Can you work these out from the model? Positions are in its coordinate system, mm. A direction names the side the tool comes from. Coordinates: 2 decimals unless noted, no trailing zeros. Order: outer loops, then holes, each group sorted by start corner. A loop starts at its lowest first (then second) coordinate and runs counter-clockwise, first axis right, second up. Notation, with made-up numbers: (11, 64.5) - (42, 64.5) arc R17 cw to (42, 93.5) - close; hole circle Ø5 at (-9, -8). An arc over 180 degrees is marked (long way). Use a Markdown table: item, result. Add a question column.
(1) I want a section at D-D (x = -2). List the corners of the cut face in (y, z) for me, and give its area (3 significant figures).
(2) I want a section at B-B (z = 1.3). List the corners of the cut face in (x, y) for me, and give its area (3 significant figures).
(3) We'd pull the mould along Y, two halves only. Please class faces 1 (the flat face through (30, 0, 2)), 2 (the cylindrical face through (-18.4, 1.2, 2.5)), 3 (the cylindrical face through (-3.45, 10.88, 2.54)): pulls with the +Y half, pulls with the -Y half, needs draft (parallel to the pull), parting line crosses it, or undercut.
(4) For pin 1 Ø5 at (x, y) = (-20, 0) entering from -Z, with a flat end and sliding along its axis, tell me the tip position at first contact or that it passes through.
(5) On a 3-axis mill with a long thin cutter (end or side, diameter ignored), from which of +Z, -Z, +X, -X, +Y, -Y can I reach the whole of each face in a straight line? I mean faces 4 (the flat face through (6, -15, 2)), 5 (the cylindrical face through (28, -19, 3)), 6 (the flat face through (6, 15, 2)). Say none if no direction works.
(6) I want a section at C-C (y = 0). List the corners of the cut face in (x, z) for me.
(7) If I drill on L1, parallel to Y at x = 20, z = 2.35; L2, parallel to X at y = -1, z = 1.2; L3, parallel to X at y = -1.5, z = 2.65, over which ranges is the centre line in solid material (lowest first)? Write a range as [from, to].
(8) I want a section at A-A (x = -20). List the corners of the cut face in (y, z) for me.
```python
from build123d import *

# Parameters (mm, degrees)
ESQUISSE1_R        = 2
BOSS_EXTRU_1_DEPTH = 5
CONG_1_R           = 5


with BuildPart() as part:
    # Esquisse1 → Boss.-Extru.1 (new body)
    with BuildSketch(Plane.XY):
        Polygon((-30, 20), (-30, -20), (-8, -20), (-4, -10), (4, -10), (8, -20), (30, -20), (30, 20), (8, 20), (4, 10), (-4, 10), (-8, 20), align=None)
        with Locations((20, 0)):
            Circle(ESQUISSE1_R, mode=Mode.SUBTRACT)
        with Locations(Location((-20, 0, 0), (0, 0, 180))):
            Circle(ESQUISSE1_R, mode=Mode.SUBTRACT)
    extrude(amount=BOSS_EXTRU_1_DEPTH)

    # Congé1
    cong_1_edges = [part.edges().sort_by_distance(p)[0] for p in [
        (-8, 20, 2.5),
        (-4, 10, 2.5),
        (4, 10, 2.5),
        (8, 20, 2.5),
        (30, 20, 2.5),
        (30, -20, 2.5),
        (8, -20, 2.5),
        (4, -10, 2.5),
        (-4, -10, 2.5),
        (-8, -20, 2.5),
        (-30, -20, 2.5),
        (-30, 20, 2.5),
    ]]
    fillet(cong_1_edges, radius=CONG_1_R)


solid = part.part
```
Answers follow:
| question | item | result |
|---|---|---|
| 1 | outline | (-10.2, 0) - (10.2, 0) - (10.2, 5) - (-10.2, 5) - close |
| 1 | area | 102 mm² |
| 2 | outline | (-30, -15) arc R5 ccw to (-25, -20) - (-11.39, -20) arc R5 ccw to (-6.74, -16.86) - (-5.26, -13.14) arc R5 cw to (-0.61, -10) - (0.61, -10) arc R5 cw to (5.26, -13.14) - (6.74, -16.86) arc R5 ccw to (11.39, -20) - (25, -20) arc R5 ccw to (30, -15) - (30, 15) arc R5 ccw to (25, 20) - (11.39, 20) arc R5 ccw to (6.74, 16.86) - (5.26, 13.14) arc R5 cw to (0.61, 10) - (-0.61, 10) arc R5 cw to (-5.26, 13.14) - (-6.74, 16.86) arc R5 ccw to (-11.39, 20) - (-25, 20) arc R5 ccw to (-30, 15) - close; hole circle Ø4 at (-20, 0); hole circle Ø4 at (20, 0) |
| 2 | area | 2,110 mm² |
| 3 | face 1 | needs draft |
| 3 | face 2 | undercut |
| 3 | face 3 | pulls with the +Y half |
| 4 | pin 1 | stops at z = 0 |
| 5 | face 4 | +Z, -Z, -Y |
| 5 | face 5 | +Z, -Z, +X, -Y |
| 5 | face 6 | +Z, -Z, +Y |
| 6 | outline | (-30, 0) - (-22, 0) - (-22, 5) - (-30, 5) - close; (-18, 0) - (18, 0) - (18, 5) - (-18, 5) - close; (22, 0) - (30, 0) - (30, 5) - (22, 5) - close |
| 7 | L1 | y = [-20, -2], [2, 20] |
| 7 | L2 | x = [-30, -21.73], [-18.27, 18.27], [21.73, 30] |
| 7 | L3 | x = [-30, -21.32], [-18.68, 18.68], [21.32, 30] |
| 8 | outline | (-20, 0) - (-2, 0) - (-2, 5) - (-20, 5) - close; (2, 0) - (20, 0) - (20, 5) - (2, 5) - close |
